Geometry check sheet. Reference: the model listing, model coordinates, mm. Coordinates: 2 decimals unless noted, no trailing zeros. Write each loop counter-clockwise with the first axis right and the second up, starting at its lowest first coordinate (ties: lowest second). Pieces come first, ordered by that corner, then holes. Notation, with made-up numbers: M 26,39.5 L 59,39.5 A22 cw 59,59.5 Z; hole C 80.25,32 d7. An arc over 180 degrees is marked long. Put each result on its own line as item: value. Start each with the question number.
1) Scan lines: line 1 along Y through (x, z) = (-13, 4); line 2 along Z through (x, y) = (32, 7). Record each from-to range of solid material in increasing order.
2) Cross-section at D-D on y = -13.5. Record the cut outline in (x, z), plus the area to 3 significant figures.
3) Cross-section at A-A on y = -3. Record the cut outline in (x, z).
4) Gauge pin test, flat ends, axial feed: pin 1 (12 mm diameter, centred on x = 21.5, y = -3.5, fed in from +Z); pin 2 (1.5 mm diameter, centred on y = 13, z = 4, fed in from -X); pin 3 (1.5 mm diameter, centred on x = -2.5, z = 6, fed in from +Y). Record the tip position at first contact, or that the pin passes through.
5) Cross-section at C-C on z = 4.25. Record the cut outline in (x, y), plus the area to 3 significant figures.
6) Cross-section at B-B on x = 5.5. Record the cut outline in (y, z), plus the area to 3 significant figures.
from build123d import *

# Parameters (mm, degrees)
F0_W     = 124
F0_H     = 40
F0_W_2   = 24
F0_H_2   = 16
F0_W_3   = 40
F0_H_3   = 2
F1_DEPTH = 2
F2_R     = 5
F3_R     = 1
F4_DEPTH = 8
F5_R     = 1


with BuildPart() as f1:
    # F0 (on Top) → F1 (new body)
    with BuildSketch(Plane.XY):
        Rectangle(F0_W, F0_H)
        Rectangle(F0_W_2, F0_H_2, mode=Mode.SUBTRACT)
        with Locations((0, 12.5)):
            Rectangle(F0_W_3, F0_H_3, mode=Mode.SUBTRACT)
    extrude(amount=F1_DEPTH)

    # F2
    f2_edges = [f1.edges().sort_by_distance(p)[0] for p in [
        (-62, 20, 1),
        (62, 20, 1),
        (62, -20, 1),
        (-62, -20, 1),
    ]]
    fillet(f2_edges, radius=F2_R)

    # F3
    f3_edges = [f1.edges().sort_by_distance(p)[0] for p in [
        (12, -8, 1),
        (-12, -8, 1),
        (12, 8, 1),
        (-12, 8, 1),
    ]]
    fillet(f3_edges, radius=F3_R)

    # F0 (on Top) → F4 (join)
    with BuildSketch(Plane.XY):
        with Locations((0, 12.5)):
            Rectangle(F0_W_3, F0_H_3)
    extrude(amount=F4_DEPTH)

    # F5
    f5_edges = [f1.edges().sort_by_distance(p)[0] for p in [
        (0, 13.5, 2),
        (20, 12.5, 8),
        (-20, 12.5, 8),
    ]]
    fillet(f5_edges, radius=F5_R)


solid = f1.part
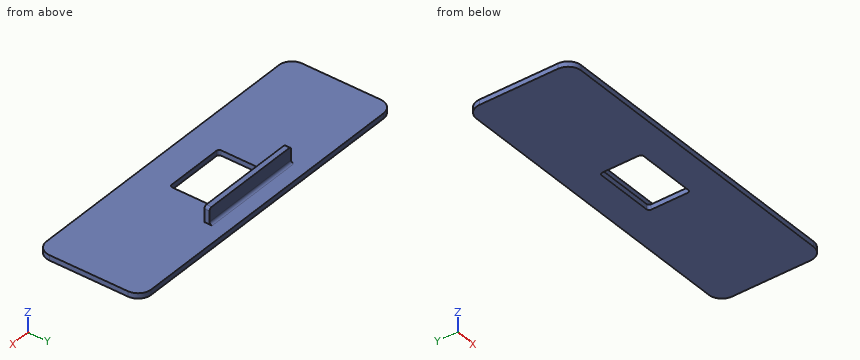
Answer key:
1. line 1: y = 11.5 to 13.5
1. line 2: z = 0 to 2
2. outline: M -62,0 L 62,0 L 62,2 L -62,2 Z
2. area: 248 mm²
3. outline: M -62,0 L -12,0 L -12,2 L -62,2 Z; M 12,0 L 62,0 L 62,2 L 12,2 Z
4. pin 1: stops at z = 2
4. pin 2: stops at x = -20
4. pin 3: stops at y = 13.5
5. outline: M -20,11.5 L 20,11.5 L 20,13.5 L -20,13.5 Z
5. area: 80.0 mm²
6. outline: M -20,0 L -8,0 L -8,2 L -20,2 Z; M 8,0 L 20,0 L 20,2 L 14.5,2 A1 cw 13.5,3 L 13.5,8 L 11.5,8 L 11.5,2 L 8,2 Z
6. area: 60.2 mm²
